For this review, take the finished solid that the model builds, in its own axes (mm). A direction names the side the tool comes from. Give positions to 0.01 mm unless a question says otherwise; leave off trailing zeros. Order: outer loops, then holes, each group sorted by start corner. A loop starts at its lowest first (then second) coordinate and runs counter-clockwise, first axis right, second up. Notation, with made-up numbers: (87.25, 3.25) - (140.25, 3.25) arc R7 cw to (140.25, 7.25) - close; hole circle Ø6 at (82.25, 35). An arc over 180 degrees is marked (long way). One line per item, written item: value.
```python
from build123d import *

# Parameters (mm, degrees)
SKETCH1_W           = 80
SKETCH1_H           = 52
SKETCH1_R           = 1.85
BOSS_EXTRUDE1_DEPTH = 1.5
SKETCH2_W           = 43.5
SKETCH2_H           = 18
BOSS_EXTRUDE2_DEPTH = 13
SKETCH3_W           = 10.5
SKETCH3_H           = 37
SKETCH3_W_2         = 50.2
SKETCH3_H_2         = 7.7
SKETCH3_W_3         = 5.5
SKETCH3_H_3         = 6.5
BOSS_EXTRUDE3_DEPTH = 11


with BuildPart() as part:
    # Sketch1 → Boss-Extrude1 (new body)
    with BuildSketch(Plane(origin=(0, 0, 0), x_dir=(1, 0, 0), z_dir=(0, 1, 0))):
        with Locations((40, 26)):
            Rectangle(SKETCH1_W, SKETCH1_H)
        with Locations(Location((3.85, 48.15, 0), (0, 0, 270))):
            Circle(SKETCH1_R, mode=Mode.SUBTRACT)
        with Locations(Location((3.85, 3.85, 0), (0, 0, 270))):
            Circle(SKETCH1_R, mode=Mode.SUBTRACT)
        with Locations(Location((76.15, 48.15, 0), (0, 0, 270))):
            Circle(SKETCH1_R, mode=Mode.SUBTRACT)
        with Locations(Location((76.15, 3.85, 0), (0, 0, 270))):
            Circle(SKETCH1_R, mode=Mode.SUBTRACT)
    extrude(amount=BOSS_EXTRUDE1_DEPTH)

    # Sketch2 → Boss-Extrude2 (add)
    with BuildSketch(Plane(origin=(0, 1.5, 0), x_dir=(1, 0, 0), z_dir=(0, 1, 0))):
        with Locations((23.75, 23)):
            Rectangle(SKETCH2_W, SKETCH2_H)
    extrude(amount=BOSS_EXTRUDE2_DEPTH)

    # Sketch3 → Boss-Extrude3 (add)
    with BuildSketch(Plane(origin=(0, 1.5, 0), x_dir=(1, 0, 0), z_dir=(0, 1, 0))):
        with Locations((62.25, 30.5)):
            Rectangle(SKETCH3_W, SKETCH3_H)
        with Locations((32.1, 7.55)):
            Rectangle(SKETCH3_W_2, SKETCH3_H_2)
        with Locations((12.45, 46.75)):
            Rectangle(SKETCH3_W_3, SKETCH3_H_3)
    extrude(amount=BOSS_EXTRUDE3_DEPTH)


solid = part.part
```
(1) Take a section at C-C (z = -40.5). Write out the cut boundary in (x, y).
Answers below:
outline: (0, 0) - (80, 0) - (80, 1.5) - (67.5, 1.5) - (67.5, 12.5) - (57, 12.5) - (57, 1.5) - (0, 1.5) - close
(2) Take a section at A-A (z = -48.15). Write out the cut boundary in (x, y).
Answers below:
outline: (0, 0) - (2, 0) - (2, 1.5) - (0, 1.5) - close; (5.7, 0) - (74.3, 0) - (74.3, 1.5) - (67.5, 1.5) - (67.5, 12.5) - (57, 12.5) - (57, 1.5) - (15.2, 1.5) - (15.2, 12.5) - (9.7, 12.5) - (9.7, 1.5) - (5.7, 1.5) - close; (78, 0) - (80, 0) - (80, 1.5) - (78, 1.5) - close
(3) Take a section at B-B (x = 3.85). Write out the cut boundary in (y, z).
Answers below:
outline: (0, -52) - (1.5, -52) - (1.5, -50) - (0, -50) - close; (0, -46.3) - (1.5, -46.3) - (1.5, -32) - (14.5, -32) - (14.5, -14) - (1.5, -14) - (1.5, -5.7) - (0, -5.7) - close; (0, -2) - (1.5, -2) - (1.5, 0) - (0, 0) - close
(4) Machinability: for faces 5 (the face through (7, 7, -7)), 6 (the face through (57.2, 7, -7)), 7 (the face through (23, 8, -14)), 8 (the face through (62, 12.5, -31)), 9 (the face through (12, 7, -50)), which of the approach directions +Z, -Z, +X, -X, +Y, -Y give a long, thin tool a straight path to every point of the face, cutting with its end or side? Answer none if there is none.
Answers below:
face 5: +Z, -X, +Y
face 6: +Z, +X, +Y
face 7: -X, +Y
face 8: +Z, -Z, +X, +Y
face 9: -Z, +X, -X, +Y
(5) Draft analysis for pull direction X (two halves, no side actions). For faces 1 (the face through (15.2, 7, -47)), 2 (the face through (32, 7, -3.7)), 3 (the face through (2, 8, -23)), 4 (the face through (77.71, 0.74, -2.855)), state which applies: pulls with the +X half, pulls with the -X half, needs draft (parallel to the pull), parting line crosses it, or undercut.
Answers below:
face 1: undercut
face 2: needs draft
face 3: pulls with the -X half
face 4: undercut
(6) Take a section at D-D (x = 63.5). Write out the cut boundary in (y, z).
Answers below:
outline: (0, -52) - (1.5, -52) - (1.5, -49) - (12.5, -49) - (12.5, -12) - (1.5, -12) - (1.5, 0) - (0, 0) - close
(7) Wall thickness on line 1 (X direction, y = 0.3, z = -48.15); line 2 (X direction, y = 11.5, z = -47); line 3 (Z direction, x = 25, y = 4.75): over which ranges is each line inside the solid? List them lowest first. Write a range as from..to.
Answers below:
line 1: x = 0..2, 5.7..74.3, 78..80
line 2: x = 9.7..15.2, 57..67.5
line 3: z = -32..-14, -11.4..-3.7
(8) For P1, Ø1.5, axis at x = 51.5, z = -7, coming from the +Y side; P2, Ø5, axis at y = 9, z = -45.5, coming from the -X side; P3, Ø4, axis at y = 11, z = -23, coming from the +X side, all flat-tipped, find the tip position at first contact; note any pin that passes through.
Answers below:
P1: stops at y = 12.5
P2: stops at x = 9.7
P3: stops at x = 67.5
